Design review of the part built by this model. Coordinates are the model's own, in mm. A direction names the side the tool comes from. Coordinates: 2 decimals unless noted, no trailing zeros. Write each loop counter-clockwise with the first axis right and the second up, starting at its lowest first coordinate (ties: lowest second). Pieces come first, ordered by that corner, then holes. Notation, with made-up numbers: M 68.5,17 L 127.5,17 A27 ccw 127.5,55 Z; hole C 40,-1.5 d9. An arc over 180 degrees is marked long. Return JSON: item names as keys, results as strings. Group by question number.
```python
from build123d import *

# Parameters (mm, degrees)
BOSS_EXTRUDE1_DEPTH     = 5
BOSS_EXTRUDE2_DEPTH     = 50
SKETCH5_R               = 3
CUT_EXTRUDE1_DEPTH      = 94.713659623
SKETCH6_R               = 5
SKETCH6_R_2             = 4
BOSS_EXTRUDE3_DEPTH     = 10
SKETCH5_3_R             = 5
SKETCH5_3_R_2           = 3
CUT_EXTRUDE2_DEPTH      = 4
ESQUISSE1_R             = 4
ENL_V_MAT_EXTRU_1_DEPTH = 100.498743711


with BuildPart() as part:
    # Sketch1 → Boss-Extrude1 (new body)
    with BuildSketch(Plane.XY):
        Polygon((43.5, -66.5), (40, -70), (0, -70), (-3.5, -66.5), (-3.5, -3.5), (0, 0), (50, 0), (50, -4), (48.5, -5.5), (43.5, -5.5), (27.557107008, -24.5), (27.557107008, -34.5), (43.5, -53.5), align=None)
    extrude(amount=BOSS_EXTRUDE1_DEPTH)

    # Sketch4 → Boss-Extrude2 (add)
    with BuildSketch(Plane(origin=(0, 0, 0), x_dir=(-1, 0, 0), z_dir=(0, 0, -1))):
        Polygon((-50, 0), (-50, -4), (-45.5, -8.5), (3.5, -8.5), (3.5, -3.5), (0, 0), align=None)
    extrude(amount=BOSS_EXTRUDE2_DEPTH)

    # Sketch5 → Cut-Extrude1 (cut, through all)
    with BuildSketch(Plane.XZ.offset(8.5)):
        with Locations(Location((32.5, -17, 0), (0, 0, 270))):
            Circle(SKETCH5_R)
        with Locations(Location((10.5, -17, 0), (0, 0, 270))):
            Circle(SKETCH5_R)
    extrude(amount=-CUT_EXTRUDE1_DEPTH, mode=Mode.SUBTRACT)

    # Sketch6 → Boss-Extrude3 (add)
    # profile 1 of 2: a face of its own
    with BuildSketch(Plane(origin=(0, 0, 0), x_dir=(-1, 0, 0), z_dir=(0, 0, -1))):
        with Locations(Location((-10, -60, 0), (0, 0, 180))):
            Circle(SKETCH6_R)
        with Locations((-10, -60)):
            Circle(SKETCH6_R_2, mode=Mode.SUBTRACT)
    # profile 2 of 2: a face of its own
    with BuildSketch(Plane(origin=(0, 0, 0), x_dir=(-1, 0, 0), z_dir=(0, 0, -1))):
        with Locations(Location((-32, -60, 0), (0, 0, 180))):
            Circle(SKETCH6_R)
        with Locations((-32, -60)):
            Circle(SKETCH6_R_2, mode=Mode.SUBTRACT)
    extrude(amount=BOSS_EXTRUDE3_DEPTH)

    # Sketch5_3 → Cut-Extrude2 (cut)
    # profile 1 of 2: a face of its own
    with BuildSketch(Plane.XZ.offset(8.5)):
        with Locations(Location((10.5, -17, 0), (0, 0, 270))):
            Circle(SKETCH5_3_R)
        with Locations(Location((10.5, -17, 0), (0, 0, 270))):
            Circle(SKETCH5_3_R_2, mode=Mode.SUBTRACT)
    # profile 2 of 2: a face of its own
    with BuildSketch(Plane.XZ.offset(8.5)):
        with Locations(Location((32.5, -17, 0), (0, 0, 270))):
            Circle(SKETCH5_3_R)
        with Locations(Location((32.5, -17, 0), (0, 0, 270))):
            Circle(SKETCH5_3_R_2, mode=Mode.SUBTRACT)
    extrude(amount=-CUT_EXTRUDE2_DEPTH, mode=Mode.SUBTRACT)

    # Esquisse1 → Enl_v. mat.-Extru.1 (cut, through all)
    with BuildSketch(Plane.XY):
        with Locations((10, -60)):
            Circle(ESQUISSE1_R)
        with Locations((32, -60)):
            Circle(ESQUISSE1_R)
    extrude(amount=ENL_V_MAT_EXTRU_1_DEPTH, mode=Mode.SUBTRACT)


solid = part.part
```
Item 1: Add section A-A (z = -17). Write out the cut boundary in (x, y), plus the area to 4 significant figures.
Item 2: The part is to be moulded in two halves that separate along Z. For faces 1 (the flat face through (15, -39, 0)), 2 (the flat face through (42, -68, 2)), 3 (the cylindrical face through (34, -6.53, -21.77)), say which applies: pulls with the +Z half, pulls with the -Z half, needs draft (parallel to the pull), parting line crosses it, or undercut.
Item 3: Add section C-C (x = 32.5). Write out the cut boundary in (y, z).
Item 4: Add section D-D (x = 39). Write out the cut boundary in (y, z).
Item 5: For line 1 (Y direction, x = 32, z = -6.75); line 2 (X direction, y = -60, z = -6.25); line 3 (X direction, y = -1.3, z = -17), list the stretches that pass through material, from the lowest coordinate up.
Item 6: For pin 1 (16 mm diameter, centred on x = 10.5, z = -17, fed in from -Y); pin 2 (4 mm diameter, centred on x = 47, z = 3, fed in from -Y); pin 3 (1.5 mm diameter, centred on y = -29, z = 2.5, fed in from +X); pin 4 (10 mm diameter, centred on x = 34.5, y = -25, fed in from -Z), all flat-tipped, find the tip position at first contact; note any pin that passes through.
Item 7: Add section B-B (y = -60). Write out the cut boundary in (x, z).
Item 8: Machinability: for faces 4 (the flat face through (18, -35, 5)), 5 (the flat face through (8, -4.5, -19)), 6 (the cylindrical face through (13, -64, -5)), 7 (the flat face through (46, -5.5, 2)), 8 (the flat face through (35.42, -43.87, 2.46)), which of the approach directions +Z, -Z, +X, -X, +Y, -Y give a long, thin tool a straight path to every point of the face, cutting with its end or side? Answer none if there is none.
Geometry check:
{
 "1": {"outline": "M -3.5,-8.5 L 5.5,-8.5 L 5.5,-4.5 L 7.5,-4.5 L 7.5,0 L 0,0 L -3.5,-3.5 Z; M 13.5,-4.5 L 15.5,-4.5 L 15.5,-8.5 L 27.5,-8.5 L 27.5,-4.5 L 29.5,-4.5 L 29.5,0 L 13.5,0 Z; M 35.5,-4.5 L 37.5,-4.5 L 37.5,-8.5 L 45.5,-8.5 L 50,-4 L 50,0 L 35.5,0 Z", "area": "304.5 mm^2"},
 "2": {"face 1": "pulls with the -Z half", "face 2": "needs draft", "face 3": "undercut"},
 "3": {"outline": "M -70,0 L -64.97,0 L -64.97,-10 L -63.97,-10 L -63.97,5 L -70,5 Z; M -56.03,-10 L -55.03,-10 L -55.03,0 L -40.39,0 L -40.39,5 L -56.03,5 Z; M -18.61,0 L -8.5,0 L -8.5,-12 L -4.5,-12 L -4.5,-14 L 0,-14 L 0,5 L -18.61,5 Z; M -8.5,-50 L 0,-50 L 0,-20 L -4.5,-20 L -4.5,-22 L -8.5,-22 Z"},
 "4": {"outline": "M -70,0 L -48.14,0 L -48.14,5 L -70,5 Z; M -10.86,0 L -8.5,0 L -8.5,-50 L 0,-50 L 0,5 L -10.86,5 Z"},
 "5": {"line 1": "-65 to -64, -56 to -55, -8.5 to 0", "line 2": "5 to 6, 14 to 15, 27 to 28, 36 to 37", "line 3": "-1.3 to 7.5, 13.5 to 29.5, 35.5 to 50"},
 "6": {"pin 1": "y = -65", "pin 2": "y = -5.5", "pin 3": "x = 27.56", "pin 4": "through"},
 "7": {"outline": "M -3.5,0 L 5,0 L 5,-10 L 6,-10 L 6,5 L -3.5,5 Z; M 14,-10 L 15,-10 L 15,0 L 27,0 L 27,-10 L 28,-10 L 28,5 L 14,5 Z; M 36,-10 L 37,-10 L 37,0 L 43.5,0 L 43.5,5 L 36,5 Z"},
 "8": {"face 4": "+Z, +X, -X, +Y, -Y", "face 5": "-Y", "face 6": "-Z", "face 7": "+Z, +X, -Y", "face 8": "+Z, -Z, +X"}
}
